```python
from build123d import *

# Parameters (mm, degrees)
BOSS_EXTRU_1_DEPTH = 191


with BuildPart() as part:
    # Esquisse1 → Boss.-Extru.1 (new body)
    with BuildSketch(Plane.XY):
        with BuildLine():
            Line((-39.529333289, 16.90370196), (-39.335219005, 16.17925759))
            ThreePointArc((-39.335219005, 16.17925759), (-18.25, 0), (-39.335219005, -16.17925759))
            Line((-39.335219005, -16.17925759), (-39.529333289, -16.90370196))
            ThreePointArc((-39.529333289, -16.90370196), (-37.17213026, -18.592337614), (-34.635254916, -19.996673749))
            ThreePointArc((-34.635254916, -19.996673749), (-34.68750182, -22.895840311), (-34.40370196, -25.781555843))
            Line((-34.40370196, -25.781555843), (-33.67925759, -25.975670127))
            ThreePointArc((-33.67925759, -25.975670127), (-9.125, -15.804963619), (-5.655961415, -42.154927717))
            Line((-5.655961415, -42.154927717), (-5.125631329, -42.685257803))
            ThreePointArc((-5.125631329, -42.685257803), (-2.48462844, -41.488177925), (0, -39.993347498))
            ThreePointArc((0, -39.993347498), (2.48462844, -41.488177925), (5.125631329, -42.685257803))
            Line((5.125631329, -42.685257803), (5.655961415, -42.154927717))
            ThreePointArc((5.655961415, -42.154927717), (9.125, -15.804963619), (33.67925759, -25.975670127))
            Line((33.67925759, -25.975670127), (34.40370196, -25.781555843))
            ThreePointArc((34.40370196, -25.781555843), (34.68750182, -22.895840311), (34.635254916, -19.996673749))
            ThreePointArc((34.635254916, -19.996673749), (37.17213026, -18.592337614), (39.529333289, -16.90370196))
            Line((39.529333289, -16.90370196), (39.335219005, -16.17925759))
            ThreePointArc((39.335219005, -16.17925759), (18.25, 0), (39.335219005, 16.17925759))
            Line((39.335219005, 16.17925759), (39.529333289, 16.90370196))
            ThreePointArc((39.529333289, 16.90370196), (37.284208364, 17.350285074), (35, 17.5))
            Line((35, 17.5), (-35, 17.5))
            ThreePointArc((-35, 17.5), (-37.284208364, 17.350285074), (-39.529333289, 16.90370196))
        make_face()
    extrude(amount=BOSS_EXTRU_1_DEPTH)


solid = part.part
```
Can you work these out from the model? Positions are in its coordinate system, mm. A direction names the side the tool comes from. Give positions to 0.01 mm unless a question says otherwise; leave off trailing zeros. Write each loop counter-clockwise with the first axis right and the second up, starting at its lowest first coordinate (ties: lowest second). Pieces come first, ordered by that corner, then holes. Notation, with made-up numbers: (48.5, 5.5) - (88.5, 5.5) arc R18 ccw to (88.5, 26.5) - close; hole circle Ø11 at (18.5, -0.5). An arc over 180 degrees is marked (long way). Write item = value, one per line. Start each with the question number.
1. Imagine slicing it at A-A (z = 113.5). Please give me the cut outline in (x, y), and give its area (3 significant figures).
2. Thinking about a two-plate mould opening in Y: for faces 1 (the face through (-1, -5, 0)), 2 (the face through (8.76, -16.02, 94.16)), 3 (the face through (-37.252, 17.354, 94.163)), which applies, released by +Y, released by -Y, zero draft, split by the parting line, or undercut?
3. Please list where these lines run through material, in increasing order: line 1 (X direction, y = -15, z = 84.5); line 2 (X direction, y = -24.5, z = 42); line 3 (Y direction, x = 24.5, z = 147).
4. Imagine slicing it at D-D (x = -16). Please give me the cut outline in (y, z), and give its area (3 significant figures).
5. Imagine slicing it at B-B (x = -3). Please give me the cut outline in (y, z).
6. On a 3-axis mill with a long thin cutter (end or side, diameter ignored), from which of +Z, -Z, +X, -X, +Y, -Y can I reach the whole of each face in a straight line? I mean faces 4 (the face through (-34.69, -22.86, 94.16)), 5 (the face through (-2.521, -41.507, 94.163)). Say none if no direction works.
7. Imagine slicing it at C-C (y = 0). Please give me the cut outline in (x, z), and give its area (3 significant figures).
8. For pin 1 (2 mm diameter, centred on x = 21.5, z = 140.5, fed in from -Y), with a flat end and sliding along its axis, tell me the tip position at first contact or that it passes through.
Worked answers:
q1.outline = (-39.53, -16.9) arc R25 ccw to (-34.64, -20) arc R25 ccw to (-34.4, -25.78) - (-33.68, -25.98) arc R16.75 cw (long way) to (-5.66, -42.15) - (-5.13, -42.69) arc R25 ccw to (0, -39.99) arc R25 ccw to (5.13, -42.69) - (5.66, -42.15) arc R16.75 cw (long way) to (33.68, -25.98) - (34.4, -25.78) arc R25 ccw to (34.64, -20) arc R25 ccw to (39.53, -16.9) - (39.34, -16.18) arc R16.75 cw (long way) to (39.34, 16.18) - (39.53, 16.9) arc R17.5 ccw to (35, 17.5) - (-35, 17.5) arc R17.5 ccw to (-39.53, 16.9) - (-39.34, 16.18) arc R16.75 cw (long way) to (-39.34, -16.18) - close
q1.area = 1,640 mm2
q2.face_1 = zero draft
q2.face_2 = undercut
q2.face_3 = released by +Y
q3.line_1 = -27.55 to -24.29, -10.71 to 10.71, 24.29 to 27.55
q3.line_2 = -34.57 to -33.21, -1.79 to 1.79, 33.21 to 34.57
q3.line_3 = -15.09 to -13.05, 13.05 to 17.5
q4.outline = (-13.63, 0) - (17.5, 0) - (17.5, 191) - (-13.63, 191) - close
q4.area = 5,950 mm2
q5.outline = (-41.75, 0) - (-38.7, 0) - (-38.7, 191) - (-41.75, 191) - close; (-21.93, 0) - (17.5, 0) - (17.5, 191) - (-21.93, 191) - close
q6.face_4 = +Z, -Z, -X
q6.face_5 = +Z, -Z, -Y
q7.outline = (-18.25, 0) - (18.25, 0) - (18.25, 191) - (-18.25, 191) - close
q7.area = 6,970 mm2
q8.pin_1 = -14.32
